Verification items for the finished model (mm, model axes). Face numbers are marked on the shaded views. Give positions to 0.01 mm unless a question says otherwise; leave off trailing zeros. Order: outer loops, then holes, each group sorted by start corner. A loop starts at its lowest first (then second) coordinate and runs counter-clockwise, first axis right, second up.
(1) Sectioned sample at C-C on y = 1. Record the cut outline in (x, z).
(2) Mould release check, pull along Y, two halves, no side actions. Record for the marked faces 1, 2 and 3: pulls with the +Y half, pulls with the -Y half, needs draft (parallel to the pull), parting line crosses it, or undercut.
(3) Gauge pin test, flat ends, axial feed: pin 1 (3 mm diameter, centred on y = 20.5, z = 2.5, fed in from -X); pin 2 (1 mm diameter, centred on y = -2.5, z = 1.5, fed in from -X). Record the tip position at first contact, or that the pin passes through.
(4) Scan lines: L1, parallel to Y at x = 0, z = 2.5; L2, parallel to Y at x = -8.5, z = 1.8; L3, parallel to X at y = -21, z = 3.85. Record each from-to range of solid material in increasing order.
(5) Sectioned sample at D-D on x = 3. Record the cut outline in (y, z), plus the area to 3 significant figures.
(6) Sectioned sample at B-B on x = 24. Record the cut outline in (y, z), plus the area to 3 significant figures.
(7) Sectioned sample at A-A on z = 3.05. Record the cut outline in (x, y), plus the area to 3 significant figures.
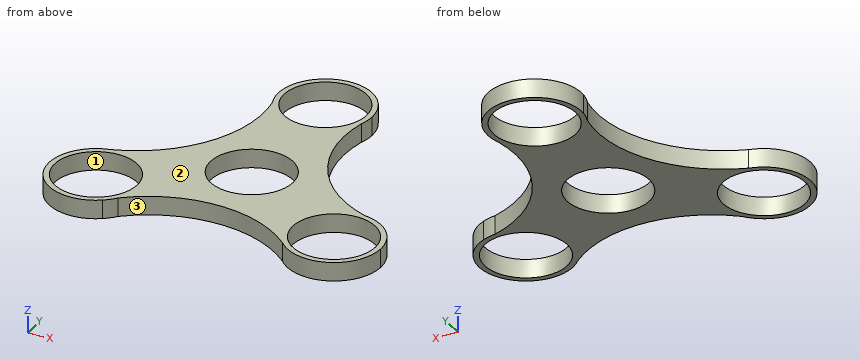
```python
from build123d import *

# Parameters (mm, degrees)
F0_R     = 11
F1_DEPTH = 5


with BuildPart() as f1:
    # F0 (on Top) → F1 (new body)
    with BuildSketch(Plane.XY):
        with BuildLine():
            ThreePointArc((11.8420038681, 32.7638646996), (12.3344040868, 34.7380581693), (12.5, 36.7659821877))
            ThreePointArc((12.5, 36.7659821877), (-0.5453664976, 49.2540795361), (-12.4524120613, 35.6762878018))
            ThreePointArc((-12.4524120613, 35.6762878018), (-11.9402706418, 33.8261206815), (-11.5348674443, 31.9496731192))
            ThreePointArc((-11.5348674443, 31.9496731192), (0.4350978948, 24.2735568899), (11.8420038681, 32.7638646996))
        make_face()
        with Locations((0, 36.7659821877)):
            Circle(F0_R, mode=Mode.SUBTRACT)
        with BuildLine():
            ThreePointArc((-11.5348674443, 31.9496731192), (-11.9402706418, 33.8261206815), (-12.4524120613, 35.6762878018))
            ThreePointArc((-12.4524120613, 35.6762878018), (-12.1375165816, 33.7775559745), (-11.5348674443, 31.9496731192))
        make_face()
        with BuildLine():
            ThreePointArc((33.436662286, -5.9853483236), (15.3144073066, 9.3071296076), (11.8420038681, 32.7638646996))
            ThreePointArc((11.8420038681, 32.7638646996), (0.4350978948, 24.2735568899), (-11.5348674443, 31.9496731192))
            ThreePointArc((-11.5348674443, 31.9496731192), (-15.7174143299, 8.6091009676), (-34.29534109, -6.1264561683))
            ThreePointArc((-34.29534109, -6.1264561683), (-23.9168388094, -8.7150458234), (-19.3402745697, -18.3829910939))
            ThreePointArc((-19.3402745697, -18.3829910939), (-19.9979564562, -22.3841786301), (-21.9017948417, -25.9643247956))
            ThreePointArc((-21.9017948417, -25.9643247956), (0.4030070232, -17.9162305753), (22.453337222, -26.6374085313))
            ThreePointArc((22.453337222, -26.6374085313), (20.8039679594, -12.513584275), (33.436662286, -5.9853483236))
        make_face()
        Circle(F0_R, mode=Mode.SUBTRACT)
        with BuildLine():
            ThreePointArc((37.1227775797, -7.0540387174), (35.2644151426, -6.5724826369), (33.436662286, -5.9853483236))
            ThreePointArc((33.436662286, -5.9853483236), (20.8039679594, -12.513584275), (22.453337222, -26.6374085313))
            ThreePointArc((22.453337222, -26.6374085313), (36.2512428961, -30.0788603828), (44.3402745697, -18.3829910939))
            ThreePointArc((44.3402745697, -18.3829910939), (42.3826008695, -11.6666411784), (37.1227775797, -7.0540387174))
        make_face()
        with Locations((31.8402745697, -18.3829910939)):
            Circle(F0_R, mode=Mode.SUBTRACT)
        with BuildLine():
            ThreePointArc((37.1227775797, -7.0540387174), (35.3209798424, -6.3773802887), (33.436662286, -5.9853483236))
            ThreePointArc((33.436662286, -5.9853483236), (35.2644151426, -6.5724826369), (37.1227775797, -7.0540387174))
        make_face()
        with BuildLine():
            ThreePointArc((-19.3402745697, -18.3829910939), (-23.9168388094, -8.7150458234), (-34.29534109, -6.1264561683))
            ThreePointArc((-34.29534109, -6.1264561683), (-43.3325593622, -23.3000420644), (-24.6703655184, -28.6222490844))
            ThreePointArc((-24.6703655184, -28.6222490844), (-23.3241445007, -27.2536380446), (-21.9017948417, -25.9643247956))
            ThreePointArc((-21.9017948417, -25.9643247956), (-19.9979564562, -22.3841786301), (-19.3402745697, -18.3829910939))
        make_face()
        with Locations((-31.8402745697, -18.3829910939)):
            Circle(F0_R, mode=Mode.SUBTRACT)
        with BuildLine():
            ThreePointArc((-21.9017948417, -25.9643247956), (-23.3241445007, -27.2536380446), (-24.6703655184, -28.6222490844))
            ThreePointArc((-24.6703655184, -28.6222490844), (-23.1834632609, -27.4001756857), (-21.9017948417, -25.9643247956))
        make_face()
    extrude(amount=F1_DEPTH)


solid = f1.part
```
Ans:
1. outline: (-21.95, 0) - (-10.95, 0) - (-10.95, 5) - (-21.95, 5) - close; (10.95, 0) - (21.85, 0) - (21.85, 5) - (10.95, 5) - close
2. face 1: undercut
2. face 2: needs draft
2. face 3: pulls with the -Y half
3. pin 1: stops at x = -11.67
3. pin 2: stops at x = -27.35
4. L1: y = -17.91 to -11, 11 to 25.77, 47.77 to 49.27
4. L2: y = -18.98 to -6.98, 6.98 to 29.78, 43.75 to 45.93
4. L3: x = -44.06 to -42.52, -21.16 to -14.16, 13.95 to 21.16, 42.52 to 44.06
5. outline: (-18.06, 0) - (-10.58, 0) - (-10.58, 5) - (-18.06, 5) - close; (10.58, 0) - (26.18, 0) - (26.18, 5) - (10.58, 5) - close; (47.35, 0) - (48.9, 0) - (48.9, 5) - (47.35, 5) - close
5. area: 123 mm2
6. outline: (-28.12, 0) - (-26.1, 0) - (-26.1, 5) - (-28.12, 5) - close; (-10.67, 0) - (-0.82, 0) - (-0.82, 5) - (-10.67, 5) - close
6. area: 59.3 mm2
7. outline: (-34.3, -6.13) arc R12.5 ccw (long way) to (-21.9, -25.96) arc R33.53 cw to (22.45, -26.64) arc R12.5 ccw (long way) to (33.44, -5.99) arc R33.53 cw to (11.84, 32.76) arc R12.5 ccw (long way) to (-11.53, 31.95) arc R33.53 cw to start; hole circle Ø22 at (-31.84, -18.38); hole circle Ø22 at (0, 0); hole circle Ø22 at (0, 36.77); hole circle Ø22 at (31.84, -18.38)
7. area: 1,660 mm2
